```python
from build123d import *

# Parameters (mm, degrees)
ESQUISSE1_R             = 28
BOSS_EXTRU_1_DEPTH      = 20
ESQUISSE2_R             = 22
ENL_V_MAT_EXTRU_1_DEPTH = 20
ESQUISSE3_R             = 28
ESQUISSE3_R_2           = 22
BOSS_EXTRU_2_DEPTH      = 30
BOSS_EXTRU_2_DRAFT      = 4


with BuildPart() as part:
    # Esquisse1 → Boss.-Extru.1 (new body)
    with BuildSketch(Plane.XY):
        Circle(ESQUISSE1_R)
    extrude(amount=BOSS_EXTRU_1_DEPTH)

    # Esquisse2 → Enlèv. mat.-Extru.1 (cut)
    with BuildSketch(Plane(origin=(0, 0, 0), x_dir=(-1, 0, 0), z_dir=(0, 0, -1))):
        Circle(ESQUISSE2_R)
    extrude(amount=-ENL_V_MAT_EXTRU_1_DEPTH, mode=Mode.SUBTRACT)


with BuildPart() as boss_extru_2_tool:
    # Esquisse3 → Boss.-Extru.2 (with draft: the straight prism first)
    with BuildSketch(Plane(origin=(0, 0, 0), x_dir=(-1, 0, 0), z_dir=(0, 0, -1))):
        Circle(ESQUISSE3_R)
        Circle(ESQUISSE3_R_2, mode=Mode.SUBTRACT)
    extrude(amount=BOSS_EXTRU_2_DEPTH)
    # Boss.-Extru.2: the draft: its side faces are tilted about the plane it starts from
    boss_extru_2_sides = [boss_extru_2_tool.faces().sort_by_distance(p)[0] for p in [
        (28, 0, -15),
        (22, 0, -15),
    ]]
    draft(boss_extru_2_sides, Plane(origin=(0, 0, 0), x_dir=(-1, 0, 0), z_dir=(0, 0, -1)), BOSS_EXTRU_2_DRAFT)


with BuildPart() as part_1:
    add(part.part)

    # Boss.-Extru.2: add boss_extru_2_tool
    add(boss_extru_2_tool.part)


solid = part_1.part
```
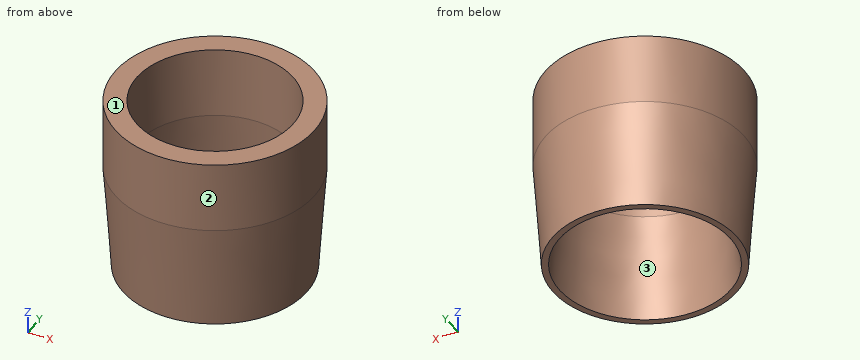
The listing builds one solid part. Answer for the finished solid, in the listing's coordinates (mm). Face numbers are marked on the shaded views. Give positions to 0.01 mm unless a question says otherwise; leave off trailing zeros. Write each loop counter-clockwise with the first axis right and the second up, starting at its lowest first coordinate (ties: lowest second). Pieces come first, ordered by that corner, then holes. Notation, with made-up numbers: (20.25, 65) - (50.25, 65) arc R26 cw to (50.25, 83) - close; hole circle Ø4 at (71.5, 82.5). An arc over 180 degrees is marked (long way). Use one line per item in the form item = value. Start each with the question number.
1) Find section A-A on x = 0. Determine the outline of the cut face in (y, z), plus the area to 3 significant figures.
2) The mould has two halves that part along X. Classify the marked faces 1, 2 and 3: pulls with the +X half, pulls with the -X half, needs draft (parallel to the pull), parting line crosses it, or undercut.
3) Find section D-D on z = -7.5. Determine the outline of the cut face in (x, y), plus the area to 3 significant figures.
4) Consider line 1 along Y through (x, z) = (-0.5, 13.5); line 2 along X through (y, z) = (8, 10.5); line 3 along Y through (x, z) = (-12.5, -18.5). Determine where each line is inside the solid, lowest interval first. Write a range as from..to.
5) Flat-ended cylindrical pins translate along their axes: pin 1 Ø5 at (x, z) = (-14.5, 5.5) entering from +Y; pin 2 Ø10 at (x, y) = (3, -15.5) entering from -Z; pin 3 Ø5 at (x, z) = (-1.5, -7.5) entering from +Y; pin 4 Ø1.5 at (y, z) = (-9.5, -23.5) entering from -X. Find the tip coordinate at first contact, or state that the pin passes through.
6) Find section C-C on z = -26. Determine the outline of the cut face in (x, y).
Geometry results:
q1.outline = (-28, 0) - (-25.9, -30) - (-24.1, -30) - (-22, 0) - (-22, 20) - (-28, 20) - close; (22, 0) - (24.1, -30) - (25.9, -30) - (28, 0) - (28, 20) - (22, 20) - close
q1.area = 474 mm2
q2.face_1 = needs draft
q2.face_2 = parting line crosses it
q2.face_3 = undercut
q3.outline = circle Ø54.95 at (0, 0); hole circle Ø45.05 at (0, 0)
q3.area = 778 mm2
q4.line_1 = -28..-21.99, 21.99..28
q4.line_2 = -26.83..-20.49, 20.49..26.83
q4.line_3 = -23.6..-19.66, 19.66..23.6
q5.pin_1 = 25.3
q5.pin_2 = through
q5.pin_3 = 27.63
q5.pin_4 = -24.87
q6.outline = circle Ø52.36 at (0, 0); hole circle Ø47.64 at (0, 0)
